Model file for the job. Use its own axes, mm. Face numbers are marked on the shaded views. A direction names the side the tool comes from. Round coordinates to 2 decimals unless told otherwise and drop trailing zeros. Order: outer loops, then holes, each group sorted by start corner. A loop starts at its lowest first (then second) coordinate and runs counter-clockwise, first axis right, second up. Notation, with made-up numbers: (64, -22) -> (123, -22) arc R5 cw to (123, -17) -> close; hole circle Ø9 at (77.25, -34.75). An arc over 180 degrees is marked (long way). Use CSV: the item, a comma, the result in double quotes.
```python
from build123d import *

# Parameters (mm, degrees)
F0_W     = 35
F0_H     = 45
F1_DEPTH = 35
F2_W     = 15
F2_H     = 4
F3_DEPTH = 6
F4_W     = 15
F4_H     = 4
F5_DEPTH = 7
F6_SIZE  = 5
F7_R     = 15
F8_DEPTH = 45.001


with BuildPart() as f1:
    # F0 (on Front) → F1 (new body)
    with BuildSketch(Plane.XZ):
        Rectangle(F0_W, F0_H)
    extrude(amount=F1_DEPTH)

    # F2 (on face) → F3 (join)
    with BuildSketch(Plane(origin=(0, 0, 0), x_dir=(-1, 0, 0), z_dir=(0, 1, 0))):
        with Locations((0, 13)):
            Rectangle(F2_W, F2_H)
    extrude(amount=F3_DEPTH)

    # F4 (on face) → F5 (join)
    with BuildSketch(Plane(origin=(0, 0, 11), x_dir=(1, 0, 0), z_dir=(0, 0, -1))):
        with Locations((0, -4)):
            Rectangle(F4_W, F4_H)
    extrude(amount=F5_DEPTH)

    # F6
    f6_edges = [f1.edges().sort_by_distance(p)[0] for p in [
        (-17.5, -35, 0),
        (17.5, -35, 0),
    ]]
    chamfer(f6_edges, length=F6_SIZE)

    # F7 (on face) → F8 (cut, through all)
    with BuildSketch(Plane.XY.offset(22.5)):
        with Locations((0, -17)):
            Circle(F7_R)
    extrude(amount=-F8_DEPTH, mode=Mode.SUBTRACT)


solid = f1.part
```
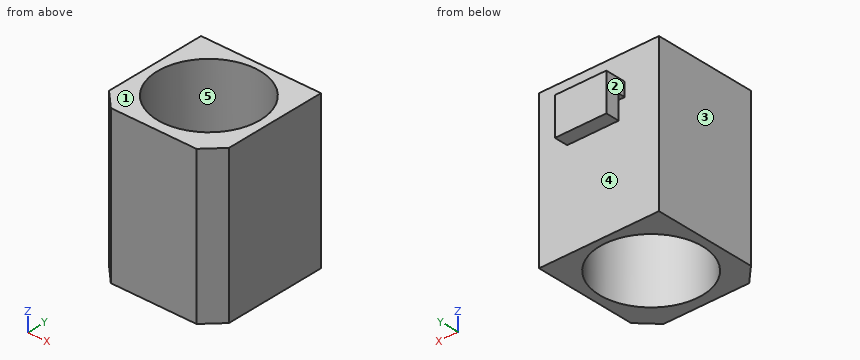
Q1. Pin check, flat tips, straight feed: pin 1 (12 mm diameter, centred on x = -4, z = -4, fed in from +Y); pin 2 (4.5 mm diameter, centred on x = -1, y = 3, fed in from -Z); pin 3 (5 mm diameter, centred on x = 2.5, y = 3.5, fed in from +Z). Stop position of each tip, or through.
From the geometry:
pin 1,"stops at y = 0"
pin 2,"stops at z = 4"
pin 3,"stops at z = 15"
Q2. Which spindle directions (+Z, -Z, +X, -X, +Y, -Y) get a long thin tool onto all of the face, cutting with end or side? Do the marked faces 1 and 2. Say none if no direction does.
From the geometry:
face 1,"+Z, +X, -X, +Y, -Y"
face 2,"+Z, -Z, -X, +Y"
Q3. Cut at D-D (z = -2.5). Give the cut face in (x, y), plus the area to 3 significant figures.
From the geometry:
outline,"(-17.5, -30) -> (-12.5, -35) -> (12.5, -35) -> (17.5, -30) -> (17.5, 0) -> (-17.5, 0) -> close; hole circle Ø30 at (0, -17)"
area,"493 mm²"
Q4. Cut at C-C (y = -17). Give the cut face in (x, z), plus the area to 3 significant figures.
From the geometry:
outline,"(-17.5, -22.5) -> (-15, -22.5) -> (-15, 22.5) -> (-17.5, 22.5) -> close; (15, -22.5) -> (17.5, -22.5) -> (17.5, 22.5) -> (15, 22.5) -> close"
area,"225 mm²"
Q5. Cut at A-A (z = 8). Give the cut face in (x, y), plus the area to 3 significant figures.
From the geometry:
outline,"(-17.5, -30) -> (-12.5, -35) -> (12.5, -35) -> (17.5, -30) -> (17.5, 0) -> (-17.5, 0) -> close; (-7.5, 2) -> (7.5, 2) -> (7.5, 6) -> (-7.5, 6) -> close; hole circle Ø30 at (0, -17)"
area,"553 mm²"
Q6. Mould opens along X. For the marked faces 3, 4 and 5 say: +X half, -X half, draft (parallel to the pull), parting line (faces both ways), or undercut.
From the geometry:
face 3,"-X half"
face 4,"draft"
face 5,"undercut"
Q7. Probe line 1 along Y through (x, z) = (0.5, -19); line 2 along Y through (x, z) = (7, -0.5); line 3 along X through (y, z) = (-24.5, -0.5). List the from-to ranges inside material, lowest first.
From the geometry:
line 1,"y = -35 to -31.99, -2.01 to 0"
line 2,"y = -35 to -30.27, -3.73 to 0"
line 3,"x = -17.5 to -12.99, 12.99 to 17.5"
Q8. Cut at B-B (x = 9). Give the cut face in (y, z).
From the geometry:
outline,"(-35, -22.5) -> (-29, -22.5) -> (-29, 22.5) -> (-35, 22.5) -> close; (-5, -22.5) -> (0, -22.5) -> (0, 22.5) -> (-5, 22.5) -> close"
